Part model, mm, in its own coordinate system. A direction names the side the tool comes from. Round coordinates to 2 decimals unless told otherwise and drop trailing zeros. Order: outer loops, then holes, each group sorted by start corner. A loop starts at its lowest first (then second) coordinate and runs counter-clockwise, first axis right, second up. Notation, with made-up numbers: (86.25, -17) -> (95.25, -17) arc R23 cw to (95.25, 9) -> close; hole circle Ø4 at (46.5, 37.5). An arc over 180 degrees is marked (long way). Return JSON: item names as keys, results as strings. Group by question number.
from build123d import *

# Parameters (mm, degrees)
SKETCH1_W           = 20
SKETCH1_H           = 254.85
BOSS_EXTRUDE1_DEPTH = 20
SKETCH3_W           = 20
SKETCH3_H           = 20
BOSS_EXTRUDE2_DEPTH = 450
SKETCH5_W           = 20
SKETCH5_H           = 20
BOSS_EXTRUDE4_DEPTH = 214.85


with BuildPart() as part:
    # Sketch1 → Boss-Extrude1 (new body)
    with BuildSketch(Plane(origin=(0, 0, 0), x_dir=(1, 0, 0), z_dir=(0, 1, 0))):
        Rectangle(SKETCH1_W, SKETCH1_H)
    extrude(amount=BOSS_EXTRUDE1_DEPTH)

    # Sketch3 → Boss-Extrude2 (add)
    with BuildSketch(Plane.ZY.offset(10)):
        with Locations((117.425, 10)):
            Rectangle(SKETCH3_W, SKETCH3_H)
        with Locations((-117.425, 10)):
            Rectangle(SKETCH3_W, SKETCH3_H)
    extrude(amount=BOSS_EXTRUDE2_DEPTH)

    # Sketch5 → Boss-Extrude4 (add)
    with BuildSketch(Plane.XY.offset(-107.425)):
        with Locations((-190, 10)):
            Rectangle(SKETCH5_W, SKETCH5_H)
    extrude(amount=BOSS_EXTRUDE4_DEPTH)


solid = part.part
(1) Mould opens along X. For faces 1 (the flat face through (10, 10, 2)), 2 (the flat face through (-180, 10, -2)), 3 (the flat face through (-228, 10, -127.425)), 4 (the flat face through (-10, 10, 2)) say: pulls with the +X half, pulls with the -X half, needs draft (parallel to the pull), parting line crosses it, or undercut.
(2) Probe L1, parallel to X at y = 15.5, z = 32.5; L2, parallel to Z at x = -440.5, y = 3.5 (3 decimals). List the from-to ranges inside material, lowest first. Write a range as [from, to].
(3) Saw through at A-A, the plane x = -235. List the corners of the cut face in (y, z) (3 decimals), and give its area (3 significant figures).
(4) Saw through at C-C, the plane y = 14.25. List the corners of the cut face in (x, z) (3 decimals).
(5) Tool access for faces 5 (the flat face through (-94, 10, 107.425)), 6 (the flat face through (-460, 10, -118)), 7 (the flat face through (-200, 10, -2)): list every direction of +Z, -Z, +X, -X, +Y, -Y with a clear straight run to the whole face (end or side of a thin tool).
(6) Pin check, flat tip, straight feed: P1, Ø10, axis at y = 6.5, z = 47, coming from the -X side. Stop position of the tip, or through.
(7) Saw through at B-B, the plane z = 40.5. List the corners of the cut face in (x, y), and give its area (3 significant figures).
Results are:
{
 "1": {"face 1": "pulls with the +X half", "face 2": "undercut", "face 3": "needs draft", "face 4": "undercut"},
 "2": {"L1": "x = [-200, -180], [-10, 10]", "L2": "z = [-127.425, -107.425], [107.425, 127.425]"},
 "3": {"outline": "(0, -127.425) -> (20, -127.425) -> (20, -107.425) -> (0, -107.425) -> close; (0, 107.425) -> (20, 107.425) -> (20, 127.425) -> (0, 127.425) -> close", "area": "800 mm^2"},
 "4": {"outline": "(-460, -127.425) -> (10, -127.425) -> (10, 127.425) -> (-460, 127.425) -> (-460, 107.425) -> (-200, 107.425) -> (-200, -107.425) -> (-460, -107.425) -> close; hole (-180, -107.425) -> (-10, -107.425) -> (-10, 107.425) -> (-180, 107.425) -> close"},
 "5": {"face 5": "+Y, -Y", "face 6": "+Z, -Z, -X, +Y, -Y", "face 7": "-X, +Y, -Y"},
 "6": {"P1": "stops at x = -200"},
 "7": {"outline": "(-200, 0) -> (-180, 0) -> (-180, 20) -> (-200, 20) -> close; (-10, 0) -> (10, 0) -> (10, 20) -> (-10, 20) -> close", "area": "800 mm^2"}
}
